The listing builds one solid part. Answer for the finished solid, in the listing's coordinates (mm). Face numbers are marked on the shaded views. Round coordinates to 2 decimals unless told otherwise and drop trailing zeros. Loops run counter-clockwise (first coordinate to the right, second up) from the corner with the lowest first, then second, coordinate; pieces in that order, holes last. Notation, with made-up numbers: (37, -27) -> (94, -27) arc R24 cw to (94, -7) -> close; hole circle Ø9 at (-22.5, -39.75). An arc over 180 degrees is marked (long way). Use a Markdown table: item, result. Add a question column.
Q1. Section B-B on y = -1.5 is taken. Give the vertices of the cut face in (x, z), then the cut area to 3 significant figures.
Q2. Consider line 1 (Y direction, x = 0.5, z = 0.6); line 2 (X direction, y = 0.5, z = 1.7); line 3 (Z direction, x = -1, y = -5). Determine where each line is inside the solid, lowest interval first.
Q3. Given pin 1 Ø4 at (x, y) = (1.5, -1.5) entering from -Z; pin 2 Ø0.6 at (x, y) = (5.66, 0.83) entering from -Z, each flat-ended and moving along its own axis, determine where each tip first touches the part or whether it passes through.
Q4. Section D-D on z = 0.25 is taken. Give the vertices of the cut face in (x, y).
Q5. Section A-A on x = 0 is taken. Give the vertices of the cut face in (y, z), then the cut area to 3 significant figures.
Q6. For a pull along Y with two mould halves and no side action, classify the marked faces 1, 2 and 3 as released by +Y, released by -Y, zero draft, split by the parting line, or undercut.
Q7. Section C-C on x = 5.66 is taken. Give the vertices of the cut face in (y, z).
from build123d import *

# Parameters (mm, degrees)
SKETCH1_W         = 20.32
SKETCH1_H         = 17.145
SKETCH1_R         = 1.397
SKETCH1_R_2       = 0.508
BOARD_DEPTH       = 2.54
SKETCH2_W         = 3
SKETCH2_H         = 6
SKETCH2_R         = 0.508
SKETCH2_R_2       = 1.008
SKETCH2_W_2       = 1.5
SKETCH2_H_2       = 0.4
SKETCH2_W_3       = 0.4
SKETCH2_H_3       = 1.389517674
SOLDER_PADS_DEPTH = 0.1


with BuildPart() as part:
    # Sketch1 → Board (new body)
    with BuildSketch(Plane.XY):
        Rectangle(SKETCH1_W, SKETCH1_H)
        with Locations((0, -6.0325)):
            Circle(SKETCH1_R, mode=Mode.SUBTRACT)
        with Locations((0, 6.0325)):
            Circle(SKETCH1_R, mode=Mode.SUBTRACT)
        with Locations((-8.66, 0.8255)):
            Circle(SKETCH1_R_2, mode=Mode.SUBTRACT)
        with Locations((8.66, 0.8255)):
            Circle(SKETCH1_R_2, mode=Mode.SUBTRACT)
        with Locations((-5.66, 0.8255)):
            Circle(SKETCH1_R_2, mode=Mode.SUBTRACT)
        with Locations((5.66, 0.8255)):
            Circle(SKETCH1_R_2, mode=Mode.SUBTRACT)
    extrude(amount=BOARD_DEPTH)

    # Sketch2 → Solder Pads (add)
    with BuildSketch(Plane.XY):
        with Locations((8.66, 0.8255)):
            Rectangle(SKETCH2_W, SKETCH2_H)
        with Locations((8.66, 0.8255)):
            Circle(SKETCH2_R, mode=Mode.SUBTRACT)
        with Locations((-8.66, 0.8255)):
            Rectangle(SKETCH2_W, SKETCH2_H)
        with Locations((-8.66, 0.8255)):
            Circle(SKETCH2_R, mode=Mode.SUBTRACT)
        with Locations((5.66, 0.8255)):
            Circle(SKETCH2_R_2)
        with Locations((5.66, 0.8255)):
            Circle(SKETCH2_R, mode=Mode.SUBTRACT)
        with Locations((-5.66, 0.8255)):
            Circle(SKETCH2_R_2)
        with Locations((-5.66, 0.8255)):
            Circle(SKETCH2_R, mode=Mode.SUBTRACT)
        with Locations((7.91, 4.7255)):
            Rectangle(SKETCH2_W_2, SKETCH2_H_2)
        with Locations((7.91, 4.732624026)):
            Rectangle(SKETCH2_W_3, SKETCH2_H_3)
        with Locations((-7.91, 4.7255)):
            Rectangle(SKETCH2_W_2, SKETCH2_H_2)
    extrude(amount=-SOLDER_PADS_DEPTH)


solid = part.part
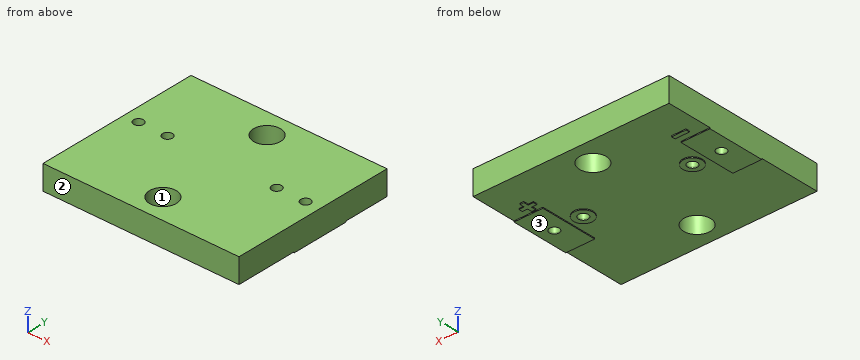
Checked values:
| question | item | result |
|---|---|---|
| 1 | outline | (-10.16, -0.1) -> (-7.16, -0.1) -> (-7.16, 0) -> (7.16, 0) -> (7.16, -0.1) -> (10.16, -0.1) -> (10.16, 2.54) -> (-10.16, 2.54) -> close |
| 1 | area | 52.2 mm2 |
| 2 | line 1 | y = -8.57 to -7.34, -4.73 to 4.73, 7.34 to 8.57 |
| 2 | line 2 | x = -10.16 to -9.05, -8.27 to -6.05, -5.27 to 5.27, 6.05 to 8.27, 9.05 to 10.16 |
| 2 | line 3 | z = 0 to 2.54 |
| 3 | pin 1 | stops at z = 0 |
| 3 | pin 2 | passes through |
| 4 | outline | (-10.16, -8.57) -> (10.16, -8.57) -> (10.16, 8.57) -> (-10.16, 8.57) -> close; hole circle Ø1.02 at (-8.66, 0.83); hole circle Ø1.02 at (-5.66, 0.83); hole circle Ø2.79 at (0, -6.03); hole circle Ø2.79 at (0, 6.03); hole circle Ø1.02 at (5.66, 0.83); hole circle Ø1.02 at (8.66, 0.83) |
| 5 | outline | (-8.57, 0) -> (-7.43, 0) -> (-7.43, 2.54) -> (-8.57, 2.54) -> close; (-4.64, 0) -> (4.64, 0) -> (4.64, 2.54) -> (-4.64, 2.54) -> close; (7.43, 0) -> (8.57, 0) -> (8.57, 2.54) -> (7.43, 2.54) -> close |
| 5 | area | 29.4 mm2 |
| 6 | face 1 | undercut |
| 6 | face 2 | released by -Y |
| 6 | face 3 | zero draft |
| 7 | outline | (-8.57, 0) -> (-0.18, 0) -> (-0.18, -0.1) -> (0.32, -0.1) -> (0.32, 2.54) -> (-8.57, 2.54) -> close; (1.33, -0.1) -> (1.83, -0.1) -> (1.83, 0) -> (8.57, 0) -> (8.57, 2.54) -> (1.33, 2.54) -> close |
